Could you check a few things on this model? Use its own coordinates, in mm. Give positions to 0.01 mm unless a question says otherwise; leave off trailing zeros. Loops run counter-clockwise (first coordinate to the right, second up) from the corner with the lowest first, then second, coordinate; pieces in that order, holes last. Notation, with made-up numbers: (73, 41) - (79, 41) arc R31 ccw to (79, 76) - close; hole circle Ø8 at (-1, 82). An arc over 180 degrees is marked (long way). Use CSV: the item, a comma, the result in double quotes.
from build123d import *


with BuildPart() as f3:
    # F0 (on Front) → F3 section 0
    with BuildSketch(Plane.XZ, mode=Mode.PRIVATE) as f3_s0:
        Polygon((-55.016788, -3.08246), (-40.163938, -37.725411), (-6.517934, -54.716223), (30.177883, -46.104706), (52.753134, -15.920285), (50.644607, 21.713415), (24.838906, 49.187166), (-12.589196, 53.645696), (-44.126672, 33.002809), align=None)
    loft([f3_s0.sketch, Vertex(0, -110, 0)])


solid = f3.part
1) We'd pull the mould along Y, two halves only. Please class faces 1 (the flat face through (-1, 0, -1)), 2 (the flat face through (22.98, -43.55, 21.22)): +Y half, -Y half, draft (parallel to the pull), parting line (faces both ways), or undercut.
Answer below:
face 1,"+Y half"
face 2,"-Y half"
2) I need wall thicknesses on line 1 along Y through (x, z) = (-43, 12); line 2 along Y through (x, z) = (-6.5, 42); line 3 along X through (y, z) = (-30.5, 21.5). Which ranges of each line are inside material? Lowest first, please.
Answer below:
line 1,"y = -15.18 to 0"
line 2,"y = -23.04 to 0"
line 3,"x = -32.6 to 31.15"
3) Suppose I cut it at B-B (y = -46.5). Please give me the cut outline in (x, z).
Answer below:
outline,"(-31.76, -1.78) - (-23.19, -21.78) - (-3.76, -31.59) - (17.42, -26.61) - (30.45, -9.19) - (29.24, 12.53) - (14.34, 28.39) - (-7.27, 30.97) - (-25.47, 19.05) - close"
4) I'm going to push flat-ended pins straight in: P1, Ø4, axis at x = 17.5, y = -23, coming from the -Z side; P2, Ø6, axis at x = -4, y = -11.5, coming from the +Z side; P3, Ø1.5, axis at y = -63, z = -13, coming from the +X side. Where does each tip first touch, or does it pass through?
Answer below:
P1,"stops at z = -39.03"
P2,"stops at z = 48.64"
P3,"stops at x = 18.62"
5) Suppose I cut it at C-C (z = -27.5). Please give me the cut outline in (x, y), plus the area to 3 significant figures.
Answer below:
outline,"(-44.55, 0) - (-29.28, -29.82) - (-3.28, -54.71) - (18, -44.39) - (44.09, 0) - close"
area,"2,960 mm2"
6) Suppose I cut it at A-A (x = -4). Please give me the cut outline in (y, z) (3 decimals).
Answer below:
outline,"(-102.002, -0.224) - (-99.045, -3.757) - (-42.494, -33.579) - (0, -54.125) - (0, 52.623) - (-75.049, 17.045) - (-100.029, 2.992) - close"
7) Suppose I cut it at D-D (y = -35). Please give me the cut outline in (x, z), plus the area to 3 significant figures.
Answer below:
outline,"(-37.51, -2.1) - (-27.38, -25.72) - (-4.44, -37.31) - (20.58, -31.44) - (35.97, -10.85) - (34.53, 14.8) - (16.94, 33.54) - (-8.58, 36.58) - (-30.09, 22.5) - close"
area,"4,080 mm2"
